The model under review builds one solid part; all positions refer to its coordinate system, in mm. A direction names the side the tool comes from. Give positions to 0.01 mm unless a question says otherwise; leave off trailing zeros. Write each loop counter-clockwise with the first axis right and the second up, starting at its lowest first coordinate (ties: lowest second). Pieces come first, ordered by that corner, then holes. Notation, with made-up numbers: (70, -29) - (87, -29) arc R15 cw to (87, -4) - close; hole circle Ø4 at (49, 87). An arc over 180 degrees is marked (long way). Write item = value, one per line.
```python
from build123d import *

# Parameters (mm, degrees)
SZKIC1_R                    = 1.5
SZKIC1_W                    = 18
SZKIC1_H                    = 44
DODANIE_WYCI_GNI_CIE1_DEPTH = 1
DODANIE_WYCI_GNI_CIE2_DEPTH = 1
DODANIE_WYCI_GNI_CIE3_DEPTH = 1
ZAOKR_GLENIE2_R             = 0.5
WYTNIJ_WYCI_GNI_CIE1_DEPTH  = 1


with BuildPart() as part:
    # Szkic1 → Dodanie-wyci_gni_cie1 (new body)
    with BuildSketch(Plane.ZY.offset(-907.5)):
        with BuildLine():
            Line((1160.348252133, 68.981105632), (1130.348252133, 95.143896329))
            Line((1130.348252133, 95.143896329), (1130.348252133, 25.4))
            ThreePointArc((1130.348252133, 25.4), (1145.348252133, 40.4), (1160.348252133, 25.4))
            Line((1160.348252133, 25.4), (1160.348252133, 68.981105632))
        make_face()
        with BuildLine():
            ThreePointArc((1160.348252133, -25.4), (1145.348252133, -40.4), (1130.348252133, -25.4))
            Line((1130.348252133, -25.4), (1130.348252133, -95.143896329))
            Line((1130.348252133, -95.143896329), (1160.348252133, -68.981105632))
            Line((1160.348252133, -68.981105632), (1160.348252133, -25.4))
        make_face()
        with BuildLine():
            ThreePointArc((1160.348252133, 25.4), (1145.348252133, 40.4), (1130.348252133, 25.4))
            Line((1130.348252133, 25.4), (1130.348252133, -25.4))
            ThreePointArc((1130.348252133, -25.4), (1145.348252133, -40.4), (1160.348252133, -25.4))
            Line((1160.348252133, -25.4), (1160.348252133, 25.4))
        make_face()
        with Locations((1145.348252133, -25.4)):
            Circle(SZKIC1_R, mode=Mode.SUBTRACT)
        with Locations((1145.348252133, 0)):
            Rectangle(SZKIC1_W, SZKIC1_H, mode=Mode.SUBTRACT)
        with Locations((1145.348252133, 25.4)):
            Circle(SZKIC1_R, mode=Mode.SUBTRACT)
    extrude(amount=DODANIE_WYCI_GNI_CIE1_DEPTH)



with BuildPart() as body_2:
    # Szkic6 → Dodanie-wyci_gni_cie2 (new body)
    with BuildSketch(Plane(origin=(0, 0, 1130.348252133), x_dir=(-1, 0, 0), z_dir=(0, 0, -1))):
        with BuildLine():
            Line((-907.5, 95.143896329), (-907.5, -95.143896329))
            add(Edge.make_bspline(
                [(-907.5, -95.143896329), (-907.5, -85.342796857), (-912.688679245, -79.610078298), (-918.5, -78.678049216)],
                knots=[0.75, 0.75, 0.75, 0.75, 0.971601315, 0.971601315, 0.971601315, 0.971601315], degree=3, weights=[0.5, 0.5, 0.630952381, 0.892857143]))
            Line((-918.5, -78.678049216), (-918.5, 78.678049216))
            add(Edge.make_bspline(
                [(-918.5, 78.678049216), (-912.688679245, 79.610078298), (-907.5, 85.342796857), (-907.5, 95.143896329)],
                knots=[0.528398685, 0.528398685, 0.528398685, 0.528398685, 0.75, 0.75, 0.75, 0.75], degree=3, weights=[0.892857143, 0.630952381, 0.5, 0.5]))
        make_face()
    extrude(amount=DODANIE_WYCI_GNI_CIE2_DEPTH)


with BuildPart() as part_1:
    add(part.part)

    add(body_2.part)  # Dodanie-wyci_gni_cie3 merges body 2
    # Szkic7 → Dodanie-wyci_gni_cie3 (add)
    with BuildSketch(Plane.ZY.offset(-907.5)):
        Polygon((1129.348252133, -95.143896329), (1129.348252133, 94.307952804), (1129.348252133, 95.143896329), (1130.348252133, 95.143896329), (1130.348252133, -95.143896329), align=None)
    extrude(amount=DODANIE_WYCI_GNI_CIE3_DEPTH)

    # Zaokr_glenie2
    zaokr_glenie2_edges = [part_1.edges().sort_by_distance(p)[0] for p in [
        (906.5, 0, 1129.348252133),
    ]]
    fillet(zaokr_glenie2_edges, radius=ZAOKR_GLENIE2_R)

    # Szkic8 → Wytnij-wyci_gni_cie1 (cut)
    with BuildSketch(Plane.ZY.offset(-906.5)):
        with BuildLine():
            ThreePointArc((1145.389561405, 40.399943118), (1151.80100132, 43.031096304), (1154.480703078, 49.422397217))
            Line((1154.480703078, 49.422397217), (1154.599387747, 73.994650155))
            Line((1154.599387747, 73.994650155), (1136.348252133, 89.91133819))
            Line((1136.348252133, 89.91133819), (1136.348252133, 49.466187083))
            ThreePointArc((1136.348252133, 49.466187083), (1138.99488175, 43.064194171), (1145.389561405, 40.399943118))
        make_face()
    wytnij_wyci_gni_cie1 = extrude(amount=-WYTNIJ_WYCI_GNI_CIE1_DEPTH, mode=Mode.SUBTRACT)

    # Lustro1: Wytnij-wyci_gni_cie1 across plane
    add(wytnij_wyci_gni_cie1.mirror(Plane.ZX), mode=Mode.SUBTRACT)


solid = part_1.part
```
1. Take a section at A-A on y = -8. Give the boundary of the cut face in (x, z).
Findings below:
outline = (906.5, 1129.85) arc R0.5 ccw to (907, 1129.35) - (918.5, 1129.35) - (918.5, 1130.35) - (907.5, 1130.35) - (907.5, 1136.35) - (906.5, 1136.35) - close; (906.5, 1154.35) - (907.5, 1154.35) - (907.5, 1160.35) - (906.5, 1160.35) - close
2. Take a section at C-C on y = 67. Give the boundary of the cut face in (x, z), and give its area (3 significant figures).
Findings below:
outline = (906.5, 1129.85) arc R0.5 ccw to (907, 1129.35) - (918.5, 1129.35) - (918.5, 1130.35) - (907.5, 1130.35) - (907.5, 1136.35) - (906.5, 1136.35) - close; (906.5, 1154.57) - (907.5, 1154.57) - (907.5, 1160.35) - (906.5, 1160.35) - close
area = 23.7 mm²
3. Take a section at D-D on z = 1132.5. Give the boundary of the cut face in (x, y).
Findings below:
outline = (906.5, -93.27) - (907.5, -93.27) - (907.5, 93.27) - (906.5, 93.27) - close
4. For line 1 (Z direction, x = 909.5, y = -45); line 2 (X direction, y = 25, z = 1155), list the stretches that pass through material, from the lowest coordinate up. Write a range as from..to.
Findings below:
line_1 = 1129.35..1130.35
line_2 = 906.5..907.5
5. Insertion check: P1, Ø6, axis at x = 914.5, y = -34, coming from the +Z side; P2, Ø4, axis at y = 25.4, z = 1145.35, coming from the +X side; P3, Ø6, axis at x = 911.5, z = 1144, coming from the -Y side. Each pin has a flat end and moves straight along its axis. Give the tip position at first contact, or say it passes through.
Findings below:
P1 = 1130.35
P2 = 907.5
P3 = through
6. Draft analysis for pull direction Z (two halves, no side actions). For faces 1 (the cylindrical face through (907.007, 24.825, 1146.734)), 2 (the flat face through (913, 1, 1129.348)), 3 (the flat face through (907.007, 71.453, 1157.514)), state which applies: +Z half, -Z half, draft (parallel to the pull), parting line (faces both ways), or undercut.
Findings below:
face_1 = undercut
face_2 = -Z half
face_3 = +Z half
7. Take a section at B-B on z = 1150.5. Give the boundary of the cut face in (x, y), and give its area (3 significant figures).
Findings below:
outline = (906.5, -41.96) - (907.5, -41.96) - (907.5, -22) - (906.5, -22) - close; (906.5, 22) - (907.5, 22) - (907.5, 41.96) - (906.5, 41.96) - close
area = 39.9 mm²
8. Machinability: for faces 4 (the flat face through (907.01, -92.56, 1133.31)), 5 (the flat face through (913, 1, 1130.348)), which of the approach directions +Z, -Z, +X, -X, +Y, -Y give a long, thin tool a straight path to every point of the face, cutting with its end or side? Answer none if there is none.
Findings below:
face_4 = +Z, +X, -X, -Y
face_5 = +Z, +X, +Y, -Y
